Can you work these out from the model? Positions are in its coordinate system, mm. A direction names the side the tool comes from. Give positions to 0.01 mm unless a question says otherwise; leave off trailing zeros. Loops run counter-clockwise (first coordinate to the right, second up) from the corner with the lowest first, then second, coordinate; pieces in that order, holes last. Notation, with made-up numbers: (52, 45) - (72, 45) arc R9 ccw to (72, 56) - close; hole circle Ø5 at (32.25, -33). An arc over 180 degrees is marked (long way). Answer as a JSON object with one key per item and string values. Group by question number.
Item 1: Which directions (+Z, -Z, +X, -X, +Y, -Y) give clear straight access to the entire face, cutting with the end or side of a thin tool? Please do faces 1 (the flat face through (-101.6, 33, 0)), 2 (the cylindrical face through (-103.25, 41.27, 0.14)).
Item 2: Suppose I cut it at C-C on y = 16.5. Write out the boundary of the cut face in (x, z), and give its area (3 significant figures).
Item 3: Suppose I cut it at A-A on z = 0. Write out the boundary of the cut face in (x, y) (3 decimals), and give its area (3 significant figures).
Item 4: Suppose I cut it at D-D on z = 14.5. Write out the boundary of the cut face in (x, y).
Item 5: Suppose I cut it at B-B on y = 38.1. Write out the boundary of the cut face in (x, z) (3 decimals).
Item 6: Please list where these lines run through material, in increasing order: L1, parallel to X at y = 36, z = -17; L2, parallel to Z at x = -103.9, y = 38.1 (3 decimals); L3, parallel to Y at x = 8, z = 1.5.
Item 7: Thinking about a two-plate mould opening in Y: for faces 3 (the cylindrical face through (103.2, 41.27, 0.14)), 4 (the flat face through (-1, 0, 0)), 5 (the flat face through (0, -2, -19.05)), which applies, pulls with the +Y half, pulls with the -Y half, needs draft (parallel to the pull), parting line crosses it, or undercut?
Item 8: Will these pins go through, and if not, where does the flat tip stop? pin 1 (12 mm diameter, centred on x = -51, z = -3, fed in from +Y); pin 2 (10 mm diameter, centred on y = 38.1, z = 0, fed in from -X).
from build123d import *

# Parameters (mm, degrees)
SKETCH1_W                      = 203.2
SKETCH1_H                      = 38.1
BASE_FLANGE1_DEPTH             = 3.2512
EDGE_FLANGE1_STRIP_W           = 14.478
EDGE_FLANGE1_STRIP_H           = 3.2512
EDGE_FLANGE1_STRIP_CUT_DEPTH   = 38.1
EDGE_FLANGE1_STRIP_2_W         = 14.478
EDGE_FLANGE1_STRIP_2_H         = 3.2512
EDGE_FLANGE1_STRIP_CUT_2_DEPTH = 38.1
EDGE_FLANGE1_DEPTH             = 38.1
EDGE_FLANGE1_BEND_DEPTH        = 38.1
SKETCH10_R                     = 3.175
CUT_EXTRUDE1_DEPTH             = 220.932373847


# Sheet-metal steps are written as plain solids
with BuildPart() as part:
    # Sketch1 → Base-Flange1 (new body)
    with BuildSketch(Plane(origin=(0, 0, 0), x_dir=(1, 0, 0), z_dir=(0, 1, 0))):
        Rectangle(SKETCH1_W, SKETCH1_H)
    extrude(amount=-BASE_FLANGE1_DEPTH)

    # Edge-Flange1 strip (across the edge) → Edge-Flange1 strip cut (cut)
    with BuildSketch(Plane(origin=(-101.6, 0, -19.05), x_dir=(1, 0, 0), z_dir=(0, 0, 1))):
        with Locations((-6.5024, -1.6256)):
            Rectangle(EDGE_FLANGE1_STRIP_W, EDGE_FLANGE1_STRIP_H)
    extrude(amount=EDGE_FLANGE1_STRIP_CUT_DEPTH, mode=Mode.SUBTRACT)

    # Edge-Flange1 strip 2 (across the edge) → Edge-Flange1 strip cut 2 (cut)
    with BuildSketch(Plane(origin=(101.6, 0, 19.05), x_dir=(-1, 0, 0), z_dir=(0, 0, -1))):
        with Locations((-6.5024, -1.6256)):
            Rectangle(EDGE_FLANGE1_STRIP_2_W, EDGE_FLANGE1_STRIP_2_H)
    extrude(amount=EDGE_FLANGE1_STRIP_CUT_2_DEPTH, mode=Mode.SUBTRACT)

    # Edge-Flange1 section (across the edge) → Edge-Flange1 (add)
    with BuildSketch(Plane(origin=(-101.6, 0, -19.05), x_dir=(1, 0, 0), z_dir=(0, 0, 1))):
        with BuildLine():
            Line((-3.2512, 0.7366), (-3.2512, 63.5))
            Line((-3.2512, 63.5), (0, 63.5))
            Line((0, 63.5), (0, 0.7366))
            ThreePointArc((0, 0.7366), (0.215745145, 0.215745145), (0.7366, 0))
            Line((0.7366, 0), (0.7366, -3.2512))
            ThreePointArc((0.7366, -3.2512), (-2.083200422, -2.083200422), (-3.2512, 0.7366))
        make_face()
    extrude(amount=EDGE_FLANGE1_DEPTH)

    # Edge-Flange1 section 2 (across the edge) → Edge-Flange1 bend (add)
    with BuildSketch(Plane(origin=(101.6, 0, 19.05), x_dir=(-1, 0, 0), z_dir=(0, 0, -1))):
        with BuildLine():
            Line((-3.2512, 0.7366), (-3.2512, 63.5))
            Line((-3.2512, 63.5), (0, 63.5))
            Line((0, 63.5), (0, 0.7366))
            ThreePointArc((0, 0.7366), (0.215745145, 0.215745145), (0.7366, 0))
            Line((0.7366, 0), (0.7366, -3.2512))
            ThreePointArc((0.7366, -3.2512), (-2.083200422, -2.083200422), (-3.2512, 0.7366))
        make_face()
    extrude(amount=EDGE_FLANGE1_BEND_DEPTH)

    # Sketch10 → Cut-Extrude1 (cut, through all)
    with BuildSketch(Plane.ZY.offset(104.8512)):
        with Locations(Location((0, 38.1, 0), (0, 0, 270))):
            Circle(SKETCH10_R)
    extrude(amount=-CUT_EXTRUDE1_DEPTH, mode=Mode.SUBTRACT)


solid = part.part
Worked out:
{
 "1": {"face 1": "+Z, -Z, +Y", "face 2": "+X, -X"},
 "2": {"outline": "(-104.85, -19.05) - (-101.6, -19.05) - (-101.6, 19.05) - (-104.85, 19.05) - close; (101.6, -19.05) - (104.85, -19.05) - (104.85, 19.05) - (101.6, 19.05) - close", "area": "248 mm2"},
 "3": {"outline": "(-104.851, 0.737) arc R3.988 ccw to (-100.863, -3.251) - (100.863, -3.251) arc R3.988 ccw to (104.851, 0.737) - (104.851, 34.925) - (101.6, 34.925) - (101.6, 0.737) arc R0.737 cw to (100.863, 0) - (-100.863, 0) arc R0.737 cw to (-101.6, 0.737) - (-101.6, 34.925) - (-104.851, 34.925) - close; (-104.851, 41.275) - (-101.6, 41.275) - (-101.6, 63.5) - (-104.851, 63.5) - close; (101.6, 41.275) - (104.851, 41.275) - (104.851, 63.5) - (101.6, 63.5) - close", "area": "1,050 mm2"},
 "4": {"outline": "(-104.85, 0.74) arc R3.99 ccw to (-100.86, -3.25) - (100.86, -3.25) arc R3.99 ccw to (104.85, 0.74) - (104.85, 63.5) - (101.6, 63.5) - (101.6, 0.74) arc R0.74 cw to (100.86, 0) - (-100.86, 0) arc R0.74 cw to (-101.6, 0.74) - (-101.6, 63.5) - (-104.85, 63.5) - close"},
 "5": {"outline": "(-104.851, -19.05) - (-101.6, -19.05) - (-101.6, -3.175) - (-104.851, -3.175) - close; (-104.851, 3.175) - (-101.6, 3.175) - (-101.6, 19.05) - (-104.851, 19.05) - close; (101.6, -19.05) - (104.851, -19.05) - (104.851, -3.175) - (101.6, -3.175) - close; (101.6, 3.175) - (104.851, 3.175) - (104.851, 19.05) - (101.6, 19.05) - close"},
 "6": {"L1": "x = -104.85 to -101.6, 101.6 to 104.85", "L2": "z = -19.05 to -3.175, 3.175 to 19.05", "L3": "y = -3.25 to 0"},
 "7": {"face 3": "undercut", "face 4": "pulls with the +Y half", "face 5": "needs draft"},
 "8": {"pin 1": "stops at y = 0", "pin 2": "stops at x = -104.85"}
}
